For this review, use the dimensioned drawing (mm, ordinates from the lowest corner) and the shaded views. Round coordinates to 2 decimals unless told otherwise and drop trailing zeros. Write each loop counter-clockwise with the first axis right and the second up, starting at its lowest first coordinate (ties: lowest second). Pieces come first, ordered by that corner, then holes. Notation, with made-up numbers: M 30.5,50.5 L 70.5,50.5 A21 ccw 70.5,73.5 Z; hole C 62,59.5 d8. An arc over 180 degrees is marked long. One line per question, with ' | ' between items.
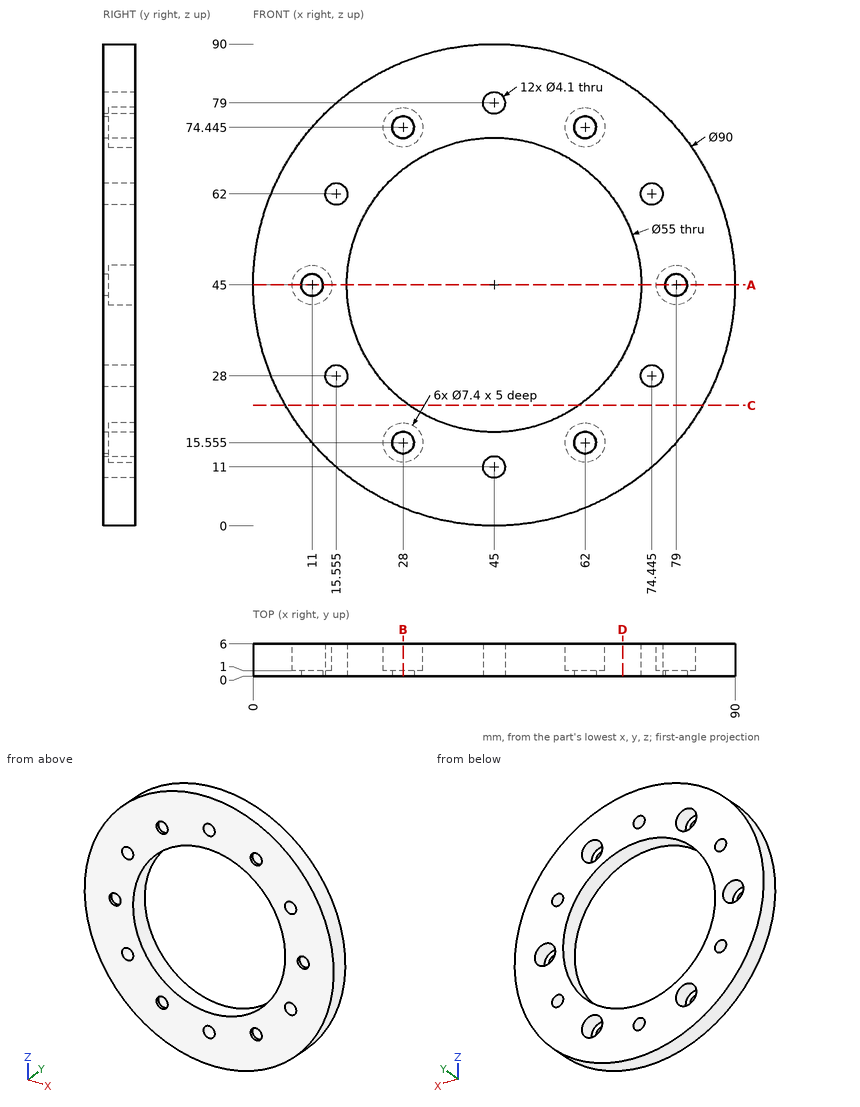
Item 1: Insertion check: pin 1 Ø1 at (y, z) = (2, 46) entering from -X; pin 2 Ø2 at (x, z) = (26.5, 74.5) entering from +Y; pin 3 Ø1 at (x, y) = (26, 1.5) entering from -Z. Each pin has a flat end and moves straight along its axis. Give the tip position at first contact, or say it passes through.
Results:
pin 1: x = 0 | pin 2: y = 1 | pin 3: z = 3.98
Item 2: Take a section at A-A (z = 45). Write out the cut boundary in (x, y), then the cut area to 3 significant figures.
Results:
outline: M 0,0 L 8.95,0 L 8.95,1 L 7.3,1 L 7.3,6 L 0,6 Z; M 13.05,0 L 17.5,0 L 17.5,6 L 14.7,6 L 14.7,1 L 13.05,1 Z; M 72.5,0 L 76.95,0 L 76.95,1 L 75.3,1 L 75.3,6 L 72.5,6 Z; M 81.05,0 L 90,0 L 90,6 L 82.7,6 L 82.7,1 L 81.05,1 Z | area: 128 mm2
Item 3: Take a section at B-B (x = 28). Write out the cut boundary in (y, z) (1 decimal), then the cut area to 3 significant figures.
Results:
outline: M 0,3.3 L 6,3.3 L 6,11.9 L 1,11.9 L 1,13.5 L 0,13.5 Z; M 0,17.6 L 1,17.6 L 1,19.3 L 6,19.3 L 6,23.4 L 0,23.4 Z; M 0,66.6 L 6,66.6 L 6,70.7 L 1,70.7 L 1,72.4 L 0,72.4 Z; M 0,76.5 L 1,76.5 L 1,78.1 L 6,78.1 L 6,86.7 L 0,86.7 Z | area: 158 mm2
Item 4: Take a section at D-D (x = 69). Write out the cut boundary in (y, z), then the cut area to 3 significant figures.
Results:
outline: M 0,6.93 L 6,6.93 L 6,31.57 L 0,31.57 Z; M 0,58.43 L 6,58.43 L 6,83.07 L 0,83.07 Z | area: 296 mm2
Item 5: To check wall thickness, follow line 1 along X through (y, z) = (3.65, 45); line 2 along X through (y, z) = (0.75, 45); line 3 along X through (y, z) = (4.7, 14.5). State the ranges of each line that lie inside material, in increasing order. Write a range as from..to.
Results:
line 1: 0..7.3, 14.7..17.5, 72.5..75.3, 82.7..90 | line 2: 0..8.95, 13.05..17.5, 72.5..76.95, 81.05..90 | line 3: 11.91..24.45, 31.55..58.45, 65.55..78.09
Item 6: Take a section at C-C (z = 22.5). Write out the cut boundary in (x, y).
Results:
outline: M 6.03,0 L 29.19,0 L 29.19,6 L 6.03,6 Z; M 60.81,0 L 83.97,0 L 83.97,6 L 60.81,6 Z
